Part model, mm, in its own coordinate system. Round coordinates to 2 decimals unless told otherwise and drop trailing zeros. Write each loop counter-clockwise with the first axis right and the second up, starting at its lowest first coordinate (ties: lowest second). Pieces come first, ordered by that corner, then holes. Notation, with made-up numbers: (77.5, -38.75) -> (114.5, -38.75) arc R13 ccw to (114.5, -13.75) -> close; hole circle Ø2 at (85, 11.25). An arc over 180 degrees is marked (long way). Return JSON: item names as keys, results as strings. Group by question number.
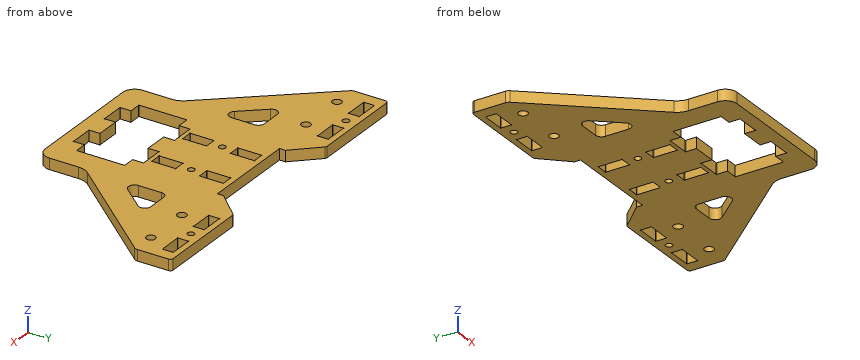
```python
from build123d import *

# Parameters (mm, degrees)
SKETCH1_R           = 2.413
SKETCH1_R_2         = 1.778
SKETCH1_W           = 12.5
SKETCH1_H           = 5.742
SKETCH1_W_2         = 51
SKETCH1_H_2         = 25.6
BOSS_EXTRUDE1_DEPTH = 5.842
FILLET1_R           = 6.35
FILLET2_R           = 3.175
FILLET3_R           = 3.175
FILLET4_R           = 1.5875
FILLET5_R           = 9.525
SKETCH2_R           = 1.778
SKETCH2_W           = 6.096
SKETCH2_H           = 12.7
CUT_EXTRUDE1_DEPTH  = 164.664917246
SKETCH3_R           = 0.1984375
CUT_EXTRUDE2_DEPTH  = 164.664917246
SKETCH5_R           = 0.1984375
CUT_EXTRUDE3_DEPTH  = 164.664917246
SKETCH9_W           = 12.7
SKETCH9_H           = 5.842
SKETCH9_W_2         = 5.842
SKETCH9_H_2         = 12.7
CUT_EXTRUDE6_DEPTH  = 164.664917246
SKETCH10_R          = 0.1984375
CUT_EXTRUDE7_DEPTH  = 164.664917246
BOSS_EXTRUDE3_DEPTH = 5.842


with BuildPart() as part:
    # Sketch1 → Boss-Extrude1 (new body)
    with BuildSketch(Plane.XY):
        Polygon((-25.4, 2.435399968), (-76.2, 2.435399968), (-76.2, 5.610399968), (-88.9, 19.1024), (-139.7, 19.1024), (-139.7, 0), (-88.9, -59.6646), (-88.9, -85.0646), (-12.7, -85.0646), (-12.7, -59.6646), (38.1, 0), (38.1, 19.1024), (-12.7, 19.1024), (-25.4, 5.610399968), align=None)
        Circle(SKETCH1_R, mode=Mode.SUBTRACT)
        with Locations((25.4, 0)):
            Circle(SKETCH1_R, mode=Mode.SUBTRACT)
        with Locations((12.7, 13.0564)):
            Circle(SKETCH1_R_2, mode=Mode.SUBTRACT)
        with Locations((-114.3, 13.0564)):
            Circle(SKETCH1_R_2, mode=Mode.SUBTRACT)
        with Locations((-127, 0)):
            Circle(SKETCH1_R, mode=Mode.SUBTRACT)
        with Locations((-101.6, 0)):
            Circle(SKETCH1_R, mode=Mode.SUBTRACT)
        with Locations((0, 13.0564)):
            Rectangle(SKETCH1_W, SKETCH1_H, mode=Mode.SUBTRACT)
        with Locations((25.4, 13.0564)):
            Rectangle(SKETCH1_W, SKETCH1_H, mode=Mode.SUBTRACT)
        with Locations((-50.8, -59.6646)):
            Rectangle(SKETCH1_W_2, SKETCH1_H_2, mode=Mode.SUBTRACT)
        Polygon((-12.7, -40.074257205), (7.882845549, -15.899705108), (-12.7, -15.899705108), align=None, mode=Mode.SUBTRACT)
        Polygon((-88.9, -15.899705108), (-109.482845549, -15.899705108), (-88.9, -40.074257205), align=None, mode=Mode.SUBTRACT)
        with Locations((-101.6, 13.0564)):
            Rectangle(SKETCH1_W, SKETCH1_H, mode=Mode.SUBTRACT)
        with Locations((-127, 13.0564)):
            Rectangle(SKETCH1_W, SKETCH1_H, mode=Mode.SUBTRACT)
    extrude(amount=BOSS_EXTRUDE1_DEPTH)

    # Fillet1
    fillet1_edges = [part.edges().sort_by_distance(p)[0] for p in [
        (-12.7, -85.0646, 2.921),
        (-88.9, -85.0646, 2.921),
    ]]
    fillet(fillet1_edges, radius=FILLET1_R)

    # Fillet2
    fillet2_edges = [part.edges().sort_by_distance(p)[0] for p in [
        (-12.7, -40.074257205, 2.921),
        (7.882845549, -15.899705108, 2.921),
        (-12.7, -15.899705108, 2.921),
        (-88.9, -15.899705108, 2.921),
        (-109.482845549, -15.899705108, 2.921),
        (-88.9, -40.074257205, 2.921),
    ]]
    fillet(fillet2_edges, radius=FILLET2_R)

    # Fillet3
    fillet3_edges = [part.edges().sort_by_distance(p)[0] for p in [
        (-139.7, 0, 2.921),
        (38.1, 0, 2.921),
    ]]
    fillet(fillet3_edges, radius=FILLET3_R)

    # Fillet4
    fillet4_edges = [part.edges().sort_by_distance(p)[0] for p in [
        (-139.7, 19.1024, 2.921),
        (-88.9, 19.1024, 2.921),
        (-12.7, 19.1024, 2.921),
        (38.1, 19.1024, 2.921),
    ]]
    fillet(fillet4_edges, radius=FILLET4_R)

    # Fillet5
    fillet5_edges = [part.edges().sort_by_distance(p)[0] for p in [
        (-88.9, -59.6646, 2.921),
        (-12.7, -59.6646, 2.921),
    ]]
    fillet(fillet5_edges, radius=FILLET5_R)

    # Sketch2 → Cut-Extrude1 (cut, through all)
    with BuildSketch(Plane.XY.offset(5.842)):
        with Locations((-38.1, -19.789600032)):
            Circle(SKETCH2_R)
        with Locations(Location((-63.5, -19.789600032, 0), (0, 0, 180))):
            Circle(SKETCH2_R)
        with Locations((-38.1, -7.089600032)):
            Rectangle(SKETCH2_W, SKETCH2_H)
        with Locations((-38.1, -32.489600032)):
            Rectangle(SKETCH2_W, SKETCH2_H)
        with Locations((-63.5, -32.489600032)):
            Rectangle(SKETCH2_W, SKETCH2_H)
        with Locations((-63.5, -7.089600032)):
            Rectangle(SKETCH2_W, SKETCH2_H)
    extrude(amount=-CUT_EXTRUDE1_DEPTH, mode=Mode.SUBTRACT)

    # Sketch3 → Cut-Extrude2 (cut, through all)
    with BuildSketch(Plane.XY.offset(5.842)):
        with Locations((-35.052, -26.139600032)):
            Circle(SKETCH3_R)
        with Locations((-41.148, -26.139600032)):
            Circle(SKETCH3_R)
        with Locations((-35.052, -38.839600032)):
            Circle(SKETCH3_R)
        with Locations((-41.148, -38.839600032)):
            Circle(SKETCH3_R)
        with Locations((-35.052, -0.739600032)):
            Circle(SKETCH3_R)
        with Locations((-35.052, -13.439600032)):
            Circle(SKETCH3_R)
        with Locations((-41.148, -13.439600032)):
            Circle(SKETCH3_R)
        with Locations((-41.148, -0.739600032)):
            Circle(SKETCH3_R)
        with Locations((-60.452, -0.739600032)):
            Circle(SKETCH3_R)
        with Locations((-60.452, -13.439600032)):
            Circle(SKETCH3_R)
        with Locations((-66.548, -13.439600032)):
            Circle(SKETCH3_R)
        with Locations((-66.548, -0.739600032)):
            Circle(SKETCH3_R)
        with Locations((-60.452, -38.839600032)):
            Circle(SKETCH3_R)
        with Locations((-66.548, -38.839600032)):
            Circle(SKETCH3_R)
        with Locations((-60.452, -26.139600032)):
            Circle(SKETCH3_R)
        with Locations((-66.548, -26.139600032)):
            Circle(SKETCH3_R)
    extrude(amount=-CUT_EXTRUDE2_DEPTH, mode=Mode.SUBTRACT)

    # Sketch5 → Cut-Extrude3 (cut, through all)
    with BuildSketch(Plane.XY.offset(5.842)):
        with Locations((31.65, 15.9274)):
            Circle(SKETCH5_R)
        with Locations((31.65, 10.1854)):
            Circle(SKETCH5_R)
        with Locations((19.15, 10.1854)):
            Circle(SKETCH5_R)
        with Locations((19.15, 15.9274)):
            Circle(SKETCH5_R)
        with Locations((6.25, 15.9274)):
            Circle(SKETCH5_R)
        with Locations((6.25, 10.1854)):
            Circle(SKETCH5_R)
        with Locations((-6.25, 15.9274)):
            Circle(SKETCH5_R)
        with Locations((-6.25, 10.1854)):
            Circle(SKETCH5_R)
        with Locations((-95.35, 10.1854)):
            Circle(SKETCH5_R)
        with Locations((-95.35, 15.9274)):
            Circle(SKETCH5_R)
        with Locations((-107.85, 10.1854)):
            Circle(SKETCH5_R)
        with Locations((-107.85, 15.9274)):
            Circle(SKETCH5_R)
        with Locations((-120.75, 15.9274)):
            Circle(SKETCH5_R)
        with Locations((-120.75, 10.1854)):
            Circle(SKETCH5_R)
        with Locations((-133.25, 10.1854)):
            Circle(SKETCH5_R)
        with Locations((-133.25, 15.9274)):
            Circle(SKETCH5_R)
        with Locations((-25.3, -46.8646)):
            Circle(SKETCH5_R)
        with Locations((-25.3, -72.4646)):
            Circle(SKETCH5_R)
        with Locations((-76.3, -72.4646)):
            Circle(SKETCH5_R)
        with Locations((-76.3, -46.8646)):
            Circle(SKETCH5_R)
    extrude(amount=-CUT_EXTRUDE3_DEPTH, mode=Mode.SUBTRACT)

    # Sketch9 → Cut-Extrude6 (cut, through all)
    with BuildSketch(Plane.XY.offset(5.842)):
        with Locations((-63.5, -43.9436)):
            Rectangle(SKETCH9_W, SKETCH9_H)
        with Locations((-38.1, -43.9436)):
            Rectangle(SKETCH9_W, SKETCH9_H)
        with Locations((-38.1, -75.3856)):
            Rectangle(SKETCH9_W, SKETCH9_H)
        with Locations((-63.5, -75.3856)):
            Rectangle(SKETCH9_W, SKETCH9_H)
        with Locations((-79.221, -59.6646)):
            Rectangle(SKETCH9_W_2, SKETCH9_H_2)
        with Locations((-22.379, -59.6646)):
            Rectangle(SKETCH9_W_2, SKETCH9_H_2)
        with Locations((-22.379, -34.2646)):
            Rectangle(SKETCH9_W_2, SKETCH9_H_2)
        with Locations((-22.379, -8.8646)):
            Rectangle(SKETCH9_W_2, SKETCH9_H_2)
        with Locations((-79.221, -8.8646)):
            Rectangle(SKETCH9_W_2, SKETCH9_H_2)
        with Locations((-79.221, -34.2646)):
            Rectangle(SKETCH9_W_2, SKETCH9_H_2)
    extrude(amount=-CUT_EXTRUDE6_DEPTH, mode=Mode.SUBTRACT)

    # Sketch10 → Cut-Extrude7 (cut, through all)
    with BuildSketch(Plane.XY.offset(5.842)):
        with Locations((-44.45, -41.0226)):
            Circle(SKETCH10_R)
        with Locations((-31.75, -41.0226)):
            Circle(SKETCH10_R)
        with Locations((-19.458, -53.3146)):
            Circle(SKETCH10_R)
        with Locations((-19.458, -66.0146)):
            Circle(SKETCH10_R)
        with Locations((-31.75, -78.3066)):
            Circle(SKETCH10_R)
        with Locations((-44.45, -78.3066)):
            Circle(SKETCH10_R)
        with Locations((-57.15, -78.3066)):
            Circle(SKETCH10_R)
        with Locations((-69.85, -78.3066)):
            Circle(SKETCH10_R)
        with Locations((-82.142, -66.0146)):
            Circle(SKETCH10_R)
        with Locations((-82.142, -53.3146)):
            Circle(SKETCH10_R)
        with Locations((-69.85, -41.0226)):
            Circle(SKETCH10_R)
        with Locations((-57.15, -41.0226)):
            Circle(SKETCH10_R)
        with Locations((-19.458, -40.6146)):
            Circle(SKETCH10_R)
        with Locations((-25.3, -40.6146)):
            Circle(SKETCH10_R)
        with Locations((-25.3, -27.9146)):
            Circle(SKETCH10_R)
        with Locations((-19.458, -27.9146)):
            Circle(SKETCH10_R)
        with Locations((-19.458, -15.2146)):
            Circle(SKETCH10_R)
        with Locations((-25.3, -15.2146)):
            Circle(SKETCH10_R)
        with Locations((-19.458, -2.5146)):
            Circle(SKETCH10_R)
        with Locations((-25.3, -2.5146)):
            Circle(SKETCH10_R)
        with Locations((-76.3, -2.5146)):
            Circle(SKETCH10_R)
        with Locations((-82.142, -2.5146)):
            Circle(SKETCH10_R)
        with Locations((-76.3, -15.2146)):
            Circle(SKETCH10_R)
        with Locations((-82.142, -15.2146)):
            Circle(SKETCH10_R)
        with Locations((-82.142, -27.9146)):
            Circle(SKETCH10_R)
        with Locations((-76.3, -27.9146)):
            Circle(SKETCH10_R)
        with Locations((-76.3, -40.6146)):
            Circle(SKETCH10_R)
        with Locations((-82.142, -40.6146)):
            Circle(SKETCH10_R)
    extrude(amount=-CUT_EXTRUDE7_DEPTH, mode=Mode.SUBTRACT)

    # Sketch11 → Boss-Extrude3 (add)
    with BuildSketch(Plane.XY.offset(5.842)):
        Polygon((-84.00501892, 0), (-76.3, 0), (-72.61548557, 0), (-72.61548557, -41.754133064), (-76.3, -41.754133064), (-76.3, -70.239806385), (-84.00501892, -70.239806385), align=None)
        Polygon((-25.3, -41.754133064), (-25.3, -70.239806385), (-17.59498108, -70.239806385), (-17.59498108, 0), (-25.3, 0), (-28.98451443, 0), (-28.98451443, -41.754133064), align=None)
    extrude(amount=-BOSS_EXTRUDE3_DEPTH)


solid = part.part
```
Item 1: Wall check: L1, parallel to X at y = -71, z = 2.8; L2, parallel to X at y = -76, z = 5.1; L3, parallel to X at y = -20, z = 1.4. Give the ranges that are in metal, low to high.
Item 2: Cut at C-C (x = -97.5). Write the cut outline in (y, z), then the cut area to 3 significant figures.
Item 3: Cut at B-B (y = -36.5). Write the cut outline in (x, z), then the cut area to 3 significant figures.
Item 4: Cut at A-A (x = -54). Write the cut outline in (y, z).
Item 5: Flat gauge pins, fed straight in: P1, Ø3, axis at y = -8.5, z = 3, coming from the +X side; P2, Ø1, axis at x = -37, z = 2, coming from the +Y side; P3, Ø3, axis at y = -15, z = 1, coming from the +X side; P4, Ø6, axis at x = -30, y = 8, coming from the -Z side. Where does each tip first touch, or does it go through?
Item 6: Cut at D-D (z = 1.85). State how many separate pieces and enclosed holes the cut face has, then the cut area to 3 significant figures.
Checks:
{
 "1": {"L1": "x = -88.9 to -76.3, -25.3 to -12.7", "L2": "x = -88.9 to -69.85, -57.15 to -44.45, -31.75 to -12.7", "L3": "x = -122.67 to -105.65, -88.9 to -65.27, -61.73 to -39.87, -36.33 to -12.7, 4.05 to 21.07"},
 "2": {"outline": "(-49.56, 0) -> (-29.97, 0) -> (-29.97, 5.84) -> (-49.56, 5.84) -> close; (-15.9, 0) -> (10.19, 0) -> (10.19, 5.84) -> (-15.9, 5.84) -> close; (15.93, 0) -> (19.1, 0) -> (19.1, 5.84) -> (15.93, 5.84) -> close", "area": "285 mm2"},
 "3": {"outline": "(-108.62, 0) -> (-66.55, 0) -> (-66.55, 5.84) -> (-108.62, 5.84) -> close; (-60.45, 0) -> (-41.15, 0) -> (-41.15, 5.84) -> (-60.45, 5.84) -> close; (-35.05, 0) -> (7.02, 0) -> (7.02, 5.84) -> (-35.05, 5.84) -> close", "area": "604 mm2"},
 "4": {"outline": "(-85.06, 0) -> (-72.46, 0) -> (-72.46, 5.84) -> (-85.06, 5.84) -> close; (-46.86, 0) -> (2.44, 0) -> (2.44, 5.84) -> (-46.86, 5.84) -> close"},
 "5": {"P1": "stops at x = 32.14", "P2": "stops at y = 2.44", "P3": "stops at x = 26.61", "P4": "passes through"},
 "6": {"separate pieces": "1", "enclosed holes": "19", "area": "9,120 mm2"}
}
